Could you check a few things on this model? Use its own coordinates, in mm. A direction names the side the tool comes from. Give positions to 0.01 mm unless a question says otherwise; leave off trailing zeros. Loops run counter-clockwise (first coordinate to the right, second up) from the corner with the lowest first, then second, coordinate; pieces in that order, holes last. Notation, with made-up numbers: (12.25, 18.25) -> (28.25, 18.25) arc R16 cw to (28.25, 44.25) -> close; hole circle Ø3 at (70.25, 0.5). An arc over 180 degrees is marked (long way). Put each result on its own line as item: value.
```python
from build123d import *

# Parameters (mm, degrees)
SKETCH1_W           = 387.4
SKETCH1_H           = 169.4
BOSS_EXTRUDE1_DEPTH = 15
SKETCH2_W           = 375.4
SKETCH2_H           = 157.4
CUT_EXTRUDE1_DEPTH  = 13
SKETCH3_W           = 40
SKETCH3_H           = 2.8
CUT_EXTRUDE2_DEPTH  = 2
BOSS_EXTRUDE2_DEPTH = 13
CUT_EXTRUDE3_DEPTH  = 212.940510521
CHAMFER1_SIZE       = 5
SKETCH7_W           = 76.032406234
SKETCH7_H           = 13
BOSS_EXTRUDE3_DEPTH = 4.323125
CHAMFER3_SIZE2      = 8.130615601
CHAMFER3_SIZE       = 4.323125
CHAMFER4_SIZE2      = 4.323125
CHAMFER4_SIZE       = 7.487872147
SKETCH8_W           = 76.032406234
SKETCH8_H           = 13
BOSS_EXTRUDE4_DEPTH = 4.323125
CHAMFER5_SIZE2      = 8.130615601
CHAMFER5_SIZE       = 4.323125
CHAMFER6_SIZE2      = 4.323125
CHAMFER6_SIZE       = 7.487872147
CUT_EXTRUDE4_DEPTH  = 2


with BuildPart() as part:
    # Sketch1 → Boss-Extrude1 (new body)
    with BuildSketch(Plane(origin=(0, 0, 0), x_dir=(1, 0, 0), z_dir=(0, 1, 0))):
        Rectangle(SKETCH1_W, SKETCH1_H)
    extrude(amount=BOSS_EXTRUDE1_DEPTH)

    # Sketch2 → Cut-Extrude1 (cut)
    with BuildSketch(Plane(origin=(0, 15, 0), x_dir=(1, 0, 0), z_dir=(0, 1, 0))):
        Rectangle(SKETCH2_W, SKETCH2_H)
    extrude(amount=-CUT_EXTRUDE1_DEPTH, mode=Mode.SUBTRACT)

    # Sketch3 → Cut-Extrude2 (cut)
    with BuildSketch(Plane(origin=(0, 15, 0), x_dir=(1, 0, 0), z_dir=(0, 1, 0))):
        with Locations((137.5, 80.1)):
            Rectangle(SKETCH3_W, SKETCH3_H)
        with Locations((-137.5, 80.1)):
            Rectangle(SKETCH3_W, SKETCH3_H)
    extrude(amount=-CUT_EXTRUDE2_DEPTH, mode=Mode.SUBTRACT)

    # Sketch4 → Boss-Extrude2 (add)
    with BuildSketch(Plane(origin=(0, 2, 0), x_dir=(1, 0, 0), z_dir=(0, 1, 0))):
        Polygon((187.7, -40.5), (105.5, -40.5), (39.760462446, -78.7), (51.702725205, -78.7), (107.116680945, -46.5), (187.7, -46.5), align=None)
        Polygon((-187.7, -46.5), (-107.116680945, -46.5), (-51.702725205, -78.7), (-39.760462446, -78.7), (-105.5, -40.5), (-187.7, -40.5), align=None)
    extrude(amount=BOSS_EXTRUDE2_DEPTH)

    # Sketch5 → Cut-Extrude3 (cut, through all)
    with BuildSketch(Plane.XZ):
        Polygon((107.116680945, 46.5), (193.7, 46.5), (193.7, 84.7), (41.377143391, 84.7), (51.702725205, 78.7), align=None)
        Polygon((-193.7, 84.7), (-193.7, 46.5), (-107.116680945, 46.5), (-51.702725205, 78.7), (-41.377143391, 84.7), align=None)
    extrude(amount=-CUT_EXTRUDE3_DEPTH, mode=Mode.SUBTRACT)

    # Chamfer1
    chamfer1_edges = [part.edges().sort_by_distance(p)[0] for p in [
        (150.408340472, 15, 46.5),
        (74.246912168, 15, 65.6),
        (-150.408340472, 15, 46.5),
        (-74.246912168, 15, 65.6),
    ]]
    chamfer(chamfer1_edges, length=CHAMFER1_SIZE)

    # Sketch7 → Boss-Extrude3 (add)
    with BuildSketch(Plane(origin=(-44.223957073, 0, 76.106347822), x_dir=(-0.8646252408638723, 0, -0.5024173492835322), z_dir=(0.5024173492835322, 0, -0.8646252408638723))):
        with Locations((32.853857148, 8.5)):
            Rectangle(SKETCH7_W, SKETCH7_H)
    extrude(amount=BOSS_EXTRUDE3_DEPTH)

    # Chamfer3
    chamfer3_edges = [part.edges().sort_by_distance(p)[0] for p in [
        (-37.588449443, 8.5, 74.962117006),
    ]]
    chamfer3_side = [part.faces().sort_by_distance(p)[0] for p in [
        (-37.631889703, 8.5, 75.036874665),
    ]]
    chamfer(chamfer3_edges, length=CHAMFER3_SIZE - 0.0001, length2=CHAMFER3_SIZE2 - 0.0001, reference=chamfer3_side[0])  # a hair under: the kernel refuses the full size

    # Chamfer4
    chamfer4_edges = [part.edges().sort_by_distance(p)[0] for p in [
        (-103.327986997, 8.5, 36.762117006),
    ]]
    chamfer4_side = [part.faces().sort_by_distance(p)[0] for p in [
        (-103.253229337, 8.5, 36.805557266),
    ]]
    chamfer(chamfer4_edges, length=CHAMFER4_SIZE - 0.0001, length2=CHAMFER4_SIZE2 - 0.0001, reference=chamfer4_side[0])  # a hair under: the kernel refuses the full size

    # Sketch8 → Boss-Extrude4 (add)
    with BuildSketch(Plane(origin=(44.223957073, 0, 76.106347822), x_dir=(-0.8646252408638638, 0, 0.5024173492835469), z_dir=(-0.5024173492835469, 0, -0.8646252408638639))):
        with Locations((-32.853857148, 8.5)):
            Rectangle(SKETCH8_W, SKETCH8_H)
    extrude(amount=BOSS_EXTRUDE4_DEPTH)

    # Chamfer5
    chamfer5_edges = [part.edges().sort_by_distance(p)[0] for p in [
        (37.588449443, 8.5, 74.962117006),
    ]]
    chamfer5_side = [part.faces().sort_by_distance(p)[0] for p in [
        (37.631889703, 8.5, 75.036874665),
    ]]
    chamfer(chamfer5_edges, length=CHAMFER5_SIZE - 0.0001, length2=CHAMFER5_SIZE2 - 0.0001, reference=chamfer5_side[0])  # a hair under: the kernel refuses the full size

    # Chamfer6
    chamfer6_edges = [part.edges().sort_by_distance(p)[0] for p in [
        (103.327986997, 8.5, 36.762117006),
    ]]
    chamfer6_side = [part.faces().sort_by_distance(p)[0] for p in [
        (103.253229337, 8.5, 36.805557266),
    ]]
    chamfer(chamfer6_edges, length=CHAMFER6_SIZE - 0.0001, length2=CHAMFER6_SIZE2 - 0.0001, reference=chamfer6_side[0])  # a hair under: the kernel refuses the full size

    # Sketch9 → Cut-Extrude4 (cut)
    with BuildSketch(Plane(origin=(0, 15, 0), x_dir=(1, 0, 0), z_dir=(0, 1, 0))):
        Polygon((70.007252271, -59.593876001), (87.472682136, -49.445045546), (85.965430137, -46.851169906), (51.034570406, -67.148830817), (52.541822405, -69.742706457), align=None)
        Polygon((-70.007251916, -59.593875391), (-87.472681782, -49.445044935), (-85.965430137, -46.851169906), (-51.034570406, -67.148830817), (-52.541822051, -69.742705846), align=None)
    extrude(amount=-CUT_EXTRUDE4_DEPTH, mode=Mode.SUBTRACT)


solid = part.part
```
1. If we section it at C-C (z = -66): List the corners of the cut face in (x, y) for me.
Recorded:
outline: (-193.7, 0) -> (193.7, 0) -> (193.7, 15) -> (187.7, 15) -> (187.7, 2) -> (-187.7, 2) -> (-187.7, 15) -> (-193.7, 15) -> close
2. If we section it at D-D (x = -81): List the corners of the cut face in (y, z) for me, then the cut area to 3 significant figures.
Recorded:
outline: (0, -84.7) -> (15, -84.7) -> (15, -78.7) -> (2, -78.7) -> (2, 49.74) -> (13, 49.74) -> (13, 53.21) -> (15, 53.21) -> (15, 55.89) -> (10, 61.68) -> (0, 61.68) -> close
area: 505 mm^2
3. I'm going to push flat-ended pins straight in: pin 1 (0.8 mm diameter, centred on x = 142.5, z = -80, fed in from +Y); pin 2 (4 mm diameter, centred on x = 47.5, y = 10, fed in from +Z); pin 3 (4 mm diameter, centred on x = -60.5, y = 10.5, fed in from +Z). Where does each tip first touch, or does it pass through?
Recorded:
pin 1: stops at y = 13
pin 2: stops at z = 82.3
pin 3: stops at z = 74.71
4. Thinking about a two-plate mould opening in X: for faces 1 (the face through (-193.7, 7, -18)), 2 (the face through (-33, 15, -80)), 3 (the face through (187.7, 9, -18)), which applies, pulls with the +X half, pulls with the -X half, needs draft (parallel to the pull), parting line crosses it, or undercut?
Recorded:
face 1: pulls with the -X half
face 2: needs draft
face 3: undercut
5. I need wall thicknesses on line 1 (X direction, y = 8, z = -20); line 2 (Z direction, x = 7.5, y = 13.25); line 3 (Z direction, x = 122, y = 7.75). Which ranges of each line are inside material? Lowest first, please.
Recorded:
line 1: x = -193.7 to -187.7, 187.7 to 193.7
line 2: z = -84.7 to -78.7, 78.7 to 84.7
line 3: z = -84.7 to -78.7, 40.5 to 46.5
6. For faces 4 (the face through (71.1, 8.59, 55.49)), 5 (the face through (193.7, 7, -18)), 6 (the face through (150, 5, 46.5)), 7 (the face through (-151, 5, 46.5)), which set-ups out of +Z, -Z, +X, -X, +Y, -Y let a thin tool reach every point of the face, with its end or its side?
Recorded:
face 4: +Y
face 5: +Z, -Z, +X, +Y, -Y
face 6: +Z, +X, +Y, -Y
face 7: +Z, -X, +Y, -Y
7. If we section it at B-B (x = -127.5): List the corners of the cut face in (y, z) for me, then the cut area to 3 significant figures.
Recorded:
outline: (0, -84.7) -> (15, -84.7) -> (15, -81.5) -> (13, -81.5) -> (13, -78.7) -> (2, -78.7) -> (2, 40.5) -> (15, 40.5) -> (15, 41.5) -> (10, 46.5) -> (0, 46.5) -> close
area: 400 mm^2
